Geometry: final body of the model. Coordinates: model frame, mm. Give positions to 0.01 mm unless a question says otherwise; leave off trailing zeros. Loops run counter-clockwise (first coordinate to the right, second up) from the corner with the lowest first, then second, coordinate; pieces in that order, holes last.
1. Section B-B, the plane x = -55. Output: boundary loops of the cut face in (y, z) (3 decimals), then the cut area to 3 significant figures.
2. Draft query along Z for faces 1 (the face through (-54.71, 1.57, 46.32)), 2 (the face through (59.1, 1.61, -49.14)), 3 (the face through (-1, 3.175, -1)). Return one class per face: +Z half, -Z half, draft (parallel to the pull), parting line (faces both ways), or undercut.
3. Section A-A, the plane z = 31. Output: boundary loops of the cut face in (x, y) (3 decimals).
4. Material intervals for line 1 along X through (y, z) = (2.2, 45); line 2 along X through (y, z) = (2.2, 31); line 3 along Z through (x, y) = (55, 1), sorted ascending.
from build123d import *

# Parameters (mm, degrees)
SKETCH1_W              = 120
SKETCH1_H              = 100
BOSS_EXTRUDE1_DEPTH    = 3.175
SKETCH2_R              = 2.794
CUT_EXTRUDE1_DEPTH     = 79.167004708
M2_5_CLEARANCE_HOLE1_D = 2.7
FILLET1_R              = 3


with BuildPart() as part:
    # Sketch1 → Boss-Extrude1 (new body)
    with BuildSketch(Plane(origin=(0, 0, 0), x_dir=(1, 0, 0), z_dir=(0, 1, 0))):
        Rectangle(SKETCH1_W, SKETCH1_H)
    extrude(amount=BOSS_EXTRUDE1_DEPTH)

    # Sketch2 → Cut-Extrude1 (cut, through all)
    with BuildSketch(Plane(origin=(0, 3.175, 0), x_dir=(1, 0, 0), z_dir=(0, 1, 0))):
        with Locations(Location((-40.75, 31, 0), (0, 0, 270))):
            Circle(SKETCH2_R)
        with Locations(Location((-40.75, -31, 0), (0, 0, 270))):
            Circle(SKETCH2_R)
        with Locations(Location((40.75, -31, 0), (0, 0, 270))):
            Circle(SKETCH2_R)
        with Locations(Location((40.75, 31, 0), (0, 0, 270))):
            Circle(SKETCH2_R)
    extrude(amount=-CUT_EXTRUDE1_DEPTH, mode=Mode.SUBTRACT)

    # M2.5 Clearance Hole1 (through all)
    with Locations(Plane(origin=(0, 3.175, 0), x_dir=(1, 0, 0), z_dir=(0, 1, 0))):
        with Locations((-55, 45), (55, 45), (-55, -45), (55, -45)):
            Hole(M2_5_CLEARANCE_HOLE1_D / 2)

    # Fillet1
    fillet1_edges = [part.edges().sort_by_distance(p)[0] for p in [
        (-60, 1.5875, -50),
        (60, 1.5875, -50),
        (60, 1.5875, 50),
        (-60, 1.5875, 50),
    ]]
    fillet(fillet1_edges, radius=FILLET1_R)


solid = part.part
Answers below:
1. outline: (0, -50) - (3.175, -50) - (3.175, -46.35) - (0, -46.35) - close; (0, -43.65) - (3.175, -43.65) - (3.175, 43.65) - (0, 43.65) - close; (0, 46.35) - (3.175, 46.35) - (3.175, 50) - (0, 50) - close
1. area: 300 mm2
2. face 1: undercut
2. face 2: -Z half
2. face 3: draft
3. outline: (-60, 0) - (-43.544, 0) - (-43.544, 3.175) - (-60, 3.175) - close; (-37.956, 0) - (37.956, 0) - (37.956, 3.175) - (-37.956, 3.175) - close; (43.544, 0) - (60, 0) - (60, 3.175) - (43.544, 3.175) - close
4. line 1: x = -60 to -56.35, -53.65 to 53.65, 56.35 to 60
4. line 2: x = -60 to -43.54, -37.96 to 37.96, 43.54 to 60
4. line 3: z = -50 to -46.35, -43.65 to 43.65, 46.35 to 50
